from build123d import *

# Parameters (mm, degrees)
F0_W     = 127
F0_H     = 101.6
F1_DEPTH = 50.8
F2_R     = 0.980775
F3_DEPTH = 2.54
F4_W     = 34.29
F4_H     = 12.7
F5_DEPTH = 6.35
F6_W     = 34.29
F6_H     = 12.7
F7_DEPTH = 6.35


with BuildPart() as f1:
    # F0 (on Top) → F1 (new body)
    with BuildSketch(Plane.XY):
        with Locations((4.771073, -7.535568)):
            Rectangle(F0_W, F0_H)
    extrude(amount=F1_DEPTH)

    # F2 (on face) → F3 (join)
    with BuildSketch(Plane.XZ.offset(58.335568)):
        with Locations((-56.460466, 2.286465)):
            Circle(F2_R)
    extrude(amount=F3_DEPTH)

    # F4 (on face) → F5 (join)
    with BuildSketch(Plane.XZ.offset(58.335568)):
        with Locations((-31.218295, 39.836608)):
            Rectangle(F4_W, F4_H)
    extrude(amount=F5_DEPTH)

    # F6 (on face) → F7 (join)
    with BuildSketch(Plane.XZ.offset(58.335568)):
        with Locations((33.035886, 39.54613)):
            Rectangle(F6_W, F6_H)
    extrude(amount=F7_DEPTH)


solid = f1.part
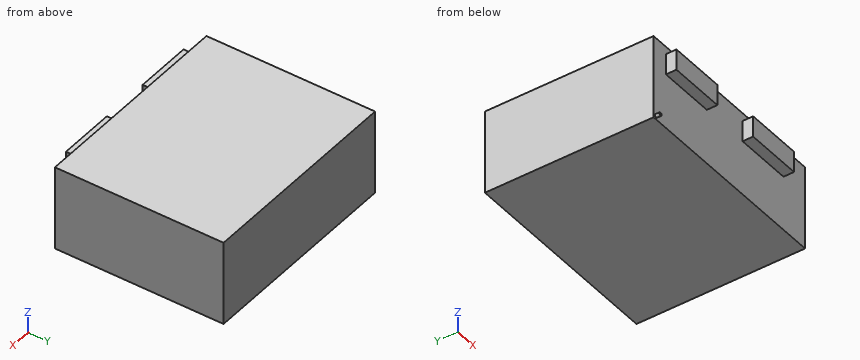
Build history of the part. All positions in model axes, mm. Coordinates: 2 decimals unless noted, no trailing zeros. Order: outer loops, then holes, each group sorted by start corner. A loop starts at its lowest first (then second) coordinate and runs counter-clockwise, first axis right, second up. Notation, with made-up numbers: (59.25, -0.5) -> (80.25, -0.5) arc R13 ccw to (80.25, 24.5) -> close; hole circle Ø8 at (32.25, 50). An arc over 180 degrees is marked (long way). One line per item, written item: value.
(1) Drop flat-ended pins along their axis: pin 1 Ø3 at (y, z) = (-61.5, 39.5) entering from -X; pin 2 Ø3 at (y, z) = (-63, 38.5) entering from +X; pin 3 Ø1.5 at (x, y) = (-42, -30.5) entering from -Z; pin 4 Ø1 at (x, z) = (-56, 2.5) entering from -Y. Give the stop position or say it passes through.
Checked values:
pin 1: x = -48.36
pin 2: x = 50.18
pin 3: z = 0
pin 4: y = -60.88
(2) Slice it at C-C, the plane x = 11.5. List the corners of the cut face in (y, z).
Checked values:
outline: (-58.34, 0) -> (43.26, 0) -> (43.26, 50.8) -> (-58.34, 50.8) -> close
(3) Slice it at B-B, the plane z = 42.5. List the corners of the cut face in (x, y), plus the area to 3 significant figures.
Checked values:
outline: (-58.73, -58.34) -> (-48.36, -58.34) -> (-48.36, -64.69) -> (-14.07, -64.69) -> (-14.07, -58.34) -> (15.89, -58.34) -> (15.89, -64.69) -> (50.18, -64.69) -> (50.18, -58.34) -> (68.27, -58.34) -> (68.27, 43.26) -> (-58.73, 43.26) -> close
area: 13,300 mm2
(4) Slice it at A-A, the plane x = 44. List the corners of the cut face in (y, z).
Checked values:
outline: (-64.69, 33.2) -> (-58.34, 33.2) -> (-58.34, 0) -> (43.26, 0) -> (43.26, 50.8) -> (-58.34, 50.8) -> (-58.34, 45.9) -> (-64.69, 45.9) -> close
(5) Slice it at D-D, the plane z = 15. List the corners of the cut face in (x, y).
Checked values:
outline: (-58.73, -58.34) -> (68.27, -58.34) -> (68.27, 43.26) -> (-58.73, 43.26) -> close
(6) Probe line 1 (Y direction, x = 16.5, z = 2). List the from-to ranges inside material, lowest first. Write a range as [from, to].
Checked values:
line 1: [-58.34, 43.26]
